Design review of the part built by this model. Coordinates are the model's own, in mm. Round coordinates to 2 decimals unless told otherwise and drop trailing zeros. Order: outer loops, then holes, each group sorted by start corner. A loop starts at its lowest first (then second) coordinate and runs counter-clockwise, first axis right, second up.
from build123d import *

# Parameters (mm, degrees)
F0_R     = 3
F1_DEPTH = 3


with BuildPart() as f1:
    # F0 (on Front) → F1 (new body)
    with BuildSketch(Plane.XZ):
        with BuildLine():
            Line((17.989963, 113.584159), (19.554308, 123.461043))
            ThreePointArc((19.554308, 123.461043), (9.807387, 124.614667), (0, 125))
            Line((0, 125), (0, 115))
            ThreePointArc((0, 115), (-9.022796, 114.645493), (-17.989963, 113.584159))
            Line((-17.989963, 113.584159), (-19.554308, 123.461043))
            ThreePointArc((-19.554308, 123.461043), (-29.18067, 121.54624), (-38.627124, 118.882065))
            Line((-38.627124, 118.882065), (-35.536954, 109.371499))
            ThreePointArc((-35.536954, 109.371499), (-44.008595, 106.246146), (-52.208907, 102.46575))
            Line((-52.208907, 102.46575), (-56.748812, 111.375816))
            ThreePointArc((-56.748812, 111.375816), (-65.312321, 106.580021), (-73.473157, 101.127124))
            Line((-73.473157, 101.127124), (-67.595304, 93.036954))
            ThreePointArc((-67.595304, 93.036954), (-74.686526, 87.446686), (-81.31728, 81.31728))
            Line((-81.31728, 81.31728), (-88.388348, 88.388348))
            ThreePointArc((-88.388348, 88.388348), (-95.050746, 81.181006), (-101.127124, 73.473157))
            Line((-101.127124, 73.473157), (-93.036954, 67.595304))
            ThreePointArc((-93.036954, 67.595304), (-98.053619, 60.087335), (-102.46575, 52.208907))
            ThreePointArc((-102.46575, 52.208907), (-106.246146, 44.008595), (-109.371499, 35.536954))
            ThreePointArc((-109.371499, 35.536954), (-111.822541, 26.846217), (-113.584159, 17.989963))
            ThreePointArc((-113.584159, 17.989963), (-114.645493, 9.022796), (-115, 0))
            ThreePointArc((-115, 0), (-114.645493, -9.022796), (-113.584159, -17.989963))
            ThreePointArc((-113.584159, -17.989963), (-111.822541, -26.846217), (-109.371499, -35.536954))
            ThreePointArc((-109.371499, -35.536954), (-106.246146, -44.008595), (-102.46575, -52.208907))
            ThreePointArc((-102.46575, -52.208907), (-98.053619, -60.087335), (-93.036954, -67.595304))
            ThreePointArc((-93.036954, -67.595304), (-87.446686, -74.686526), (-81.31728, -81.31728))
            ThreePointArc((-81.31728, -81.31728), (-74.686526, -87.446686), (-67.595304, -93.036954))
            ThreePointArc((-67.595304, -93.036954), (-60.087335, -98.053619), (-52.208907, -102.46575))
            ThreePointArc((-52.208907, -102.46575), (-44.008595, -106.246146), (-35.536954, -109.371499))
            ThreePointArc((-35.536954, -109.371499), (-26.846217, -111.822541), (-17.989963, -113.584159))
            ThreePointArc((-17.989963, -113.584159), (-9.022796, -114.645493), (0, -115))
            ThreePointArc((0, -115), (9.022796, -114.645493), (17.989963, -113.584159))
            ThreePointArc((17.989963, -113.584159), (26.846217, -111.822541), (35.536954, -109.371499))
            ThreePointArc((35.536954, -109.371499), (44.008595, -106.246146), (52.208907, -102.46575))
            ThreePointArc((52.208907, -102.46575), (60.087335, -98.053619), (67.595304, -93.036954))
            ThreePointArc((67.595304, -93.036954), (74.686526, -87.446686), (81.31728, -81.31728))
            ThreePointArc((81.31728, -81.31728), (87.446686, -74.686526), (93.036954, -67.595304))
            ThreePointArc((93.036954, -67.595304), (98.053619, -60.087335), (102.46575, -52.208907))
            ThreePointArc((102.46575, -52.208907), (106.246146, -44.008595), (109.371499, -35.536954))
            ThreePointArc((109.371499, -35.536954), (111.822541, -26.846217), (113.584159, -17.989963))
            ThreePointArc((113.584159, -17.989963), (114.645493, -9.022796), (115, 0))
            ThreePointArc((115, 0), (114.645493, 9.022796), (113.584159, 17.989963))
            ThreePointArc((113.584159, 17.989963), (111.822541, 26.846217), (109.371499, 35.536954))
            ThreePointArc((109.371499, 35.536954), (106.246146, 44.008595), (102.46575, 52.208907))
            ThreePointArc((102.46575, 52.208907), (98.053619, 60.087335), (93.036954, 67.595304))
            ThreePointArc((93.036954, 67.595304), (87.446686, 74.686526), (81.31728, 81.31728))
            ThreePointArc((81.31728, 81.31728), (74.686526, 87.446686), (67.595304, 93.036954))
            ThreePointArc((67.595304, 93.036954), (60.087335, 98.053619), (52.208907, 102.46575))
            Line((52.208907, 102.46575), (56.748812, 111.375816))
            ThreePointArc((56.748812, 111.375816), (47.835429, 115.484942), (38.627124, 118.882065))
            Line((38.627124, 118.882065), (35.536954, 109.371499))
            ThreePointArc((35.536954, 109.371499), (26.846217, 111.822541), (17.989963, 113.584159))
        make_face()
        with Locations((-85.932023, 51.143791)):
            Circle(F0_R, mode=Mode.SUBTRACT)
        with BuildLine():
            ThreePointArc((0.469303, 2.963065), (2.281218, 1.948344), (3, 0))
            ThreePointArc((3, 0), (-2.12132, -2.12132), (0, 3))
            ThreePointArc((0, 3), (0.235377, 2.990752), (0.469303, 2.963065))
        make_face(mode=Mode.SUBTRACT)
        with BuildLine():
            Line((73.473157, 101.127124), (67.595304, 93.036954))
            ThreePointArc((67.595304, 93.036954), (74.686526, 87.446686), (81.31728, 81.31728))
            Line((81.31728, 81.31728), (88.388348, 88.388348))
            ThreePointArc((88.388348, 88.388348), (81.181006, 95.050746), (73.473157, 101.127124))
        make_face()
        with BuildLine():
            Line((101.127124, 73.473157), (93.036954, 67.595304))
            ThreePointArc((93.036954, 67.595304), (98.053619, 60.087335), (102.46575, 52.208907))
            Line((102.46575, 52.208907), (111.375816, 56.748812))
            ThreePointArc((111.375816, 56.748812), (106.580021, 65.312321), (101.127124, 73.473157))
        make_face()
        with BuildLine():
            Line((118.882065, 38.627124), (109.371499, 35.536954))
            ThreePointArc((109.371499, 35.536954), (111.822541, 26.846217), (113.584159, 17.989963))
            Line((113.584159, 17.989963), (123.461043, 19.554308))
            ThreePointArc((123.461043, 19.554308), (121.54624, 29.18067), (118.882065, 38.627124))
        make_face()
        with BuildLine():
            Line((125, 0), (115, 0))
            ThreePointArc((115, 0), (114.645493, -9.022796), (113.584159, -17.989963))
            Line((113.584159, -17.989963), (123.461043, -19.554308))
            ThreePointArc((123.461043, -19.554308), (124.614667, -9.807387), (125, 0))
        make_face()
        with BuildLine():
            Line((118.882065, -38.627124), (109.371499, -35.536954))
            ThreePointArc((109.371499, -35.536954), (106.246146, -44.008595), (102.46575, -52.208907))
            Line((102.46575, -52.208907), (111.375816, -56.748812))
            ThreePointArc((111.375816, -56.748812), (115.484942, -47.835429), (118.882065, -38.627124))
        make_face()
        with BuildLine():
            ThreePointArc((-109.371499, 35.536954), (-106.246146, 44.008595), (-102.46575, 52.208907))
            Line((-102.46575, 52.208907), (-111.375816, 56.748812))
            ThreePointArc((-111.375816, 56.748812), (-115.484942, 47.835429), (-118.882065, 38.627124))
            Line((-118.882065, 38.627124), (-109.371499, 35.536954))
        make_face()
        with BuildLine():
            Line((101.127124, -73.473157), (93.036954, -67.595304))
            ThreePointArc((93.036954, -67.595304), (87.446686, -74.686526), (81.31728, -81.31728))
            Line((81.31728, -81.31728), (88.388348, -88.388348))
            ThreePointArc((88.388348, -88.388348), (95.050746, -81.181006), (101.127124, -73.473157))
        make_face()
        with BuildLine():
            ThreePointArc((-115, 0), (-114.645493, 9.022796), (-113.584159, 17.989963))
            Line((-113.584159, 17.989963), (-123.461043, 19.554308))
            ThreePointArc((-123.461043, 19.554308), (-124.614667, 9.807387), (-125, 0))
            Line((-125, 0), (-115, 0))
        make_face()
        with BuildLine():
            Line((73.473157, -101.127124), (67.595304, -93.036954))
            ThreePointArc((67.595304, -93.036954), (60.087335, -98.053619), (52.208907, -102.46575))
            Line((52.208907, -102.46575), (56.748812, -111.375816))
            ThreePointArc((56.748812, -111.375816), (65.312321, -106.580021), (73.473157, -101.127124))
        make_face()
        with BuildLine():
            ThreePointArc((-109.371499, -35.536954), (-111.822541, -26.846217), (-113.584159, -17.989963))
            Line((-113.584159, -17.989963), (-123.461043, -19.554308))
            ThreePointArc((-123.461043, -19.554308), (-121.54624, -29.18067), (-118.882065, -38.627124))
            Line((-118.882065, -38.627124), (-109.371499, -35.536954))
        make_face()
        with BuildLine():
            Line((38.627124, -118.882065), (35.536954, -109.371499))
            ThreePointArc((35.536954, -109.371499), (26.846217, -111.822541), (17.989963, -113.584159))
            Line((17.989963, -113.584159), (19.554308, -123.461043))
            ThreePointArc((19.554308, -123.461043), (29.18067, -121.54624), (38.627124, -118.882065))
        make_face()
        with BuildLine():
            ThreePointArc((-93.036954, -67.595304), (-98.053619, -60.087335), (-102.46575, -52.208907))
            Line((-102.46575, -52.208907), (-111.375816, -56.748812))
            ThreePointArc((-111.375816, -56.748812), (-106.580021, -65.312321), (-101.127124, -73.473157))
            Line((-101.127124, -73.473157), (-93.036954, -67.595304))
        make_face()
        with BuildLine():
            Line((0, -125), (0, -115))
            ThreePointArc((0, -115), (-9.022796, -114.645493), (-17.989963, -113.584159))
            Line((-17.989963, -113.584159), (-19.554308, -123.461043))
            ThreePointArc((-19.554308, -123.461043), (-9.807387, -124.614667), (0, -125))
        make_face()
        with BuildLine():
            ThreePointArc((-67.595304, -93.036954), (-74.686526, -87.446686), (-81.31728, -81.31728))
            Line((-81.31728, -81.31728), (-88.388348, -88.388348))
            ThreePointArc((-88.388348, -88.388348), (-81.181006, -95.050746), (-73.473157, -101.127124))
            Line((-73.473157, -101.127124), (-67.595304, -93.036954))
        make_face()
        with BuildLine():
            Line((-38.627124, -118.882065), (-35.536954, -109.371499))
            ThreePointArc((-35.536954, -109.371499), (-44.008595, -106.246146), (-52.208907, -102.46575))
            Line((-52.208907, -102.46575), (-56.748812, -111.375816))
            ThreePointArc((-56.748812, -111.375816), (-47.835429, -115.484942), (-38.627124, -118.882065))
        make_face()
    extrude(amount=F1_DEPTH)


solid = f1.part
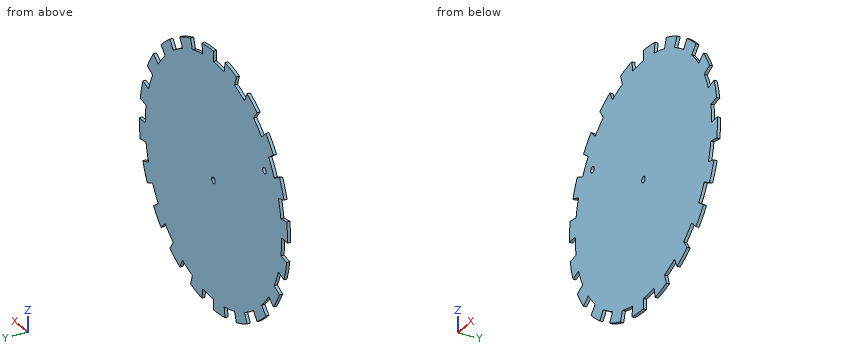
1) To check wall thickness, follow line 1 along Z through (x, y) = (68.5, -2.45); line 2 along Z through (x, y) = (56.5, -2.6); line 3 along X through (y, z) = (-2.2, 49.5). State the ranges of each line that lie inside material, in increasing order.
Results:
line 1: z = -104.56 to -94.28, -92.37 to 94.28
line 2: z = -110.89 to 100.16, 110.89 to 111.5
line 3: x = -114.78 to -88.44, -83.42 to 103.8
2) Take a section at A-A on y = -1.95. State how many separate pieces and enclosed holes the cut face has, plus the area to 3 significant figures.
Results:
separate pieces: 1
enclosed holes: 2
area: 45,300 mm2
3) Take a section at B-B on x = -62. Give the boundary of the cut face in (y, z).
Results:
outline: (-3, -96.86) - (0, -96.86) - (0, 108.54) - (-3, 108.54) - close
4) Clearance check with a flat-ended pin moving along its axis: P1, Ø1.5, axis at x = 43.5, y = -2, coming from the -Z side. State where the tip first meets the part, or that it passes through.
Results:
P1: stops at z = -106.76
